```python
from build123d import *

# Parameters (mm, degrees)
BOSS_EXTRUDE1_START     = 13.5
BOSS_EXTRUDE1_DEPTH     = 7
BOSS_EXTRUDE2_START     = 20.5
SKETCH2_W               = 8
SKETCH2_H               = 6
BOSS_EXTRUDE2_DEPTH     = 6
CUT_EXTRUDE1_DEPTH      = 39.389329572
CUT_EXTRUDE1_DEPTH_BACK = 39.389329572
SKETCH3_R               = 0.9
CUT_EXTRUDE2_DEPTH      = 39.389329572
CUT_EXTRUDE2_DEPTH_BACK = 39.389329572
SKETCH4_W               = 8
SKETCH4_H               = 2.4
CUT_EXTRUDE3_DEPTH      = 39.389329572
CUT_EXTRUDE3_DEPTH_BACK = 39.389329572
SKETCH5_R               = 1.2


with BuildPart() as part:
    # Sketch1 → Boss-Extrude1 (new body)
    with BuildSketch(Plane.XY.offset(BOSS_EXTRUDE1_START)):
        Polygon((-16.7, 19.975), (19.3, 19.975), (19.3, 13.975), (17.125805621, 13.975), (15.988398639, 10.85), (14.642129734, 10.85), (13.504722752, 13.975), (12.41341664, 13.975), (11.276009658, 10.85), (9.929740754, 10.85), (8.792333772, 13.975), (7.70102766, 13.975), (6.563620678, 10.85), (5.217351773, 10.85), (4.079944791, 13.975), (2.988638679, 13.975), (1.851231697, 10.85), (0.504962793, 10.85), (-0.632444189, 13.975), (-1.723750301, 13.975), (-2.861157283, 10.85), (-4.207426188, 10.85), (-5.34483317, 13.975), (-6.436139281, 13.975), (-7.573546263, 10.85), (-8.919815168, 10.85), (-10.05722215, 13.975), (-16.7, 13.975), align=None)
    extrude(amount=BOSS_EXTRUDE1_DEPTH)

    # Sketch2 → Boss-Extrude2 (add)
    with BuildSketch(Plane.XY.offset(BOSS_EXTRUDE2_START)):
        with Locations((15.3, 16.975)):
            Rectangle(SKETCH2_W, SKETCH2_H)
    extrude(amount=BOSS_EXTRUDE2_DEPTH)

    # Sketch3 → Cut-Extrude1 (cut, two sides: drawn at the far end of the back side and taken through both)
    with BuildSketch(Plane(origin=(0, 0, 0), x_dir=(1, 0, 0), z_dir=(0, 1, 0)).offset(-CUT_EXTRUDE1_DEPTH_BACK)):
        with Locations(Location((17.8, -24.5, 0), (0, 0, 270))):
            Circle(SKETCH3_R)
    extrude(amount=CUT_EXTRUDE1_DEPTH + CUT_EXTRUDE1_DEPTH_BACK, mode=Mode.SUBTRACT)

    # Sketch4 → Cut-Extrude2 (cut, two sides: drawn at the far end of the back side and taken through both)
    with BuildSketch(Plane.XY.offset(-CUT_EXTRUDE2_DEPTH_BACK)):
        with Locations((-7.7, 16.975)):
            Rectangle(SKETCH4_W, SKETCH4_H)
    extrude(amount=CUT_EXTRUDE2_DEPTH + CUT_EXTRUDE2_DEPTH_BACK, mode=Mode.SUBTRACT)

    # Sketch5 → Cut-Extrude3 (cut, two sides: drawn at the far end of the back side and taken through both)
    with BuildSketch(Plane.XY.offset(-CUT_EXTRUDE3_DEPTH_BACK)):
        with Locations((-11.7, 16.975)):
            Circle(SKETCH5_R)
        with Locations((-3.7, 16.975)):
            Circle(SKETCH5_R)
    extrude(amount=CUT_EXTRUDE3_DEPTH + CUT_EXTRUDE3_DEPTH_BACK, mode=Mode.SUBTRACT)


solid = part.part
```
Check sheet for the modelled part. Datum: model origin and axes. Units: mm. A direction names the side the tool comes from. Round coordinates to 2 decimals unless told otherwise and drop trailing zeros. Loops run counter-clockwise (first coordinate to the right, second up) from the corner with the lowest first, then second, coordinate; pieces in that order, holes last. Notation, with made-up numbers: (24, -3.75) - (71, -3.75) arc R37 cw to (71, 35.25) - close; hole circle Ø9 at (66, 30.5). An arc over 180 degrees is marked (long way). Answer as a JSON object with one key per item and string values. Group by question number.
Q1. Sectioned sample at B-B, the plane y = 17.5. Enter the section's corners in (x, z), plus the area to 3 significant figures.
Q2. Sectioned sample at D-D, the plane z = 24.5. Enter the section's corners in (x, y) (3 decimals), plus the area to 3 significant figures.
Q3. Mould release check, pull along Y, two halves, no side actions. Record for faces 4 (the face through (11.85, 12.43, 16.95)), 5 (the face through (11.3, 17, 23)), 6 (the face through (-2.5, 16.95, 16.95)): released by +Y, released by -Y, zero draft, split by the parting line, or undercut.
Q4. Gauge pin test, flat ends, axial feed: P1, Ø1, axis at y = 17.5, z = 24, coming from the -X side; P2, Ø0.5, axis at x = 8.5, z = 17.5, coming from the -Y side (3 decimals); P3, Ø4.5, axis at x = 0.5, y = 13.5, coming from the +Z side. Record the tip position at first contact, or that the pin passes through.
Q5. Scan lines: line 1 along X through (y, z) = (18.75, 24.5); line 2 along Y through (x, z) = (-4, 15) (3 decimals); line 3 along Z through (x, y) = (17.8, 17.5). Record each from-to range of solid material in increasing order. Write a range as [from, to].
Q6. Set-up check for faces 1 (the face through (-1, 13.975, 17)), 2 (the face through (15, 13.975, 21)), 3 (the face through (15, 10.85, 17)): record each of +Z, -Z, +X, -X, +Y, -Y from which the full face is reachable in a straight line by a thin tool's end or side.
Q7. Sectioned sample at A-A, the plane x = 17.8. Enter the section's corners in (y, z) (3 decimals), plus the area to 3 significant figures.
Solution:
{
 "1": {"outline": "(-16.7, 13.5) - (-12.78, 13.5) - (-12.78, 20.5) - (-16.7, 20.5) - close; (-2.62, 13.5) - (19.3, 13.5) - (19.3, 26.5) - (11.3, 26.5) - (11.3, 20.5) - (-2.62, 20.5) - close; hole circle Ø1.8 at (17.8, 24.5)", "area": "226 mm²"},
 "2": {"outline": "(11.3, 13.975) - (16.9, 13.975) - (16.9, 19.975) - (11.3, 19.975) - close; (18.7, 13.975) - (19.3, 13.975) - (19.3, 19.975) - (18.7, 19.975) - close", "area": "37.2 mm²"},
 "3": {"face 4": "released by -Y", "face 5": "zero draft", "face 6": "undercut"},
 "4": {"P1": "stops at x = 11.3", "P2": "stops at y = 13.975", "P3": "stops at z = 20.5"},
 "5": {"line 1": "x = [11.3, 16.9], [18.7, 19.3]", "line 2": "y = [10.85, 15.775], [18.175, 19.975]", "line 3": "z = [13.5, 23.6], [25.4, 26.5]"},
 "6": {"face 1": "+Z, -Z, -Y", "face 2": "+Z, -Y", "face 3": "+Z, -Z, +X, -X, -Y"},
 "7": {"outline": "(13.975, 13.5) - (19.975, 13.5) - (19.975, 23.6) - (13.975, 23.6) - close; (13.975, 25.4) - (19.975, 25.4) - (19.975, 26.5) - (13.975, 26.5) - close", "area": "67.2 mm²"}
}
